The listing builds one solid part. Answer for the finished solid, in the listing's coordinates (mm). Give positions to 0.01 mm unless a question says otherwise; leave off trailing zeros. Order: outer loops, then holes, each group sorted by start corner. A loop starts at its lowest first (then second) coordinate and runs counter-clockwise, first axis right, second up.
```python
from build123d import *

# Parameters (mm, degrees)
SKETCH1_R           = 1.5875
BOSS_EXTRUDE1_DEPTH = 18.25625


with BuildPart() as part:
    # Sketch1 → Boss-Extrude1 (new body)
    with BuildSketch(Plane.XY):
        with BuildLine():
            Line((0, 990.6), (0, 0))
            Line((0, 0), (457.201, 0))
            Line((457.201, 0), (457.201, 13.862038208))
            ThreePointArc((457.201, 13.862038208), (232.767577124, 176.628269142), (124.367415652, 431.8))
            Line((124.367415652, 431.8), (50.8, 990.6))
            Line((50.8, 990.6), (0, 990.6))
        make_face()
        with Locations((18.25625, 18.25625)):
            Circle(SKETCH1_R, mode=Mode.SUBTRACT)
        with Locations((18.25625, 43.65625)):
            Circle(SKETCH1_R, mode=Mode.SUBTRACT)
        with Locations((56.35625, 63.5)):
            Circle(SKETCH1_R, mode=Mode.SUBTRACT)
        with Locations((56.35625, 101.6)):
            Circle(SKETCH1_R, mode=Mode.SUBTRACT)
        with Locations((388.14375, 18.25625)):
            Circle(SKETCH1_R, mode=Mode.SUBTRACT)
        with Locations((18.25625, 972.34375)):
            Circle(SKETCH1_R, mode=Mode.SUBTRACT)
    extrude(amount=BOSS_EXTRUDE1_DEPTH)


solid = part.part
```
1) Find section B-B (y = 498.5). Write down the section's boundary in (x, z).
Geometry says:
outline: (0, 0) - (115.59, 0) - (115.59, 18.26) - (0, 18.26) - close
2) Straight lines are drawn through the part: probe 1 along Y at (x, z) = (246, 10); probe 2 along Y at (x, z) = (256, 16.75); probe 3 along X at (y, z) = (425.5, 4.75). For each, find the intervals that lie inside material, in ascending order.
Geometry says:
probe 1: y = 0 to 160.68
probe 2: y = 0 to 149.44
probe 3: x = 0 to 125.24
3) Given P1, Ø3, axis at x = 18.26, y = 972.34, coming from the -Z side; P2, Ø6, axis at y = 548.5, z = 12.5, coming from the +X side; P3, Ø4, axis at x = 224, z = 12.5, coming from the +Y side; P4, Ø1, axis at y = 326.5, z = 7.5, coming from the +X side, each flat-ended and moving along its own axis, determine where each tip first touches the part or whether it passes through.
Geometry says:
P1: passes through
P2: stops at x = 109.4
P3: stops at y = 190.63
P4: stops at x = 149.82
4) Find section C-C (x = 165). Write down the section's boundary in (y, z), then the cut area to 3 significant figures.
Geometry says:
outline: (0, 0) - (288.08, 0) - (288.08, 18.26) - (0, 18.26) - close
area: 5,260 mm2
5) Find section A-A (z = 7). Write down the section's boundary in (x, y) (1 decimal).
Geometry says:
outline: (0, 0) - (457.2, 0) - (457.2, 13.9) arc R518.2 cw to (124.4, 431.8) - (50.8, 990.6) - (0, 990.6) - close; hole circle Ø3.2 at (18.3, 18.3); hole circle Ø3.2 at (18.3, 43.7); hole circle Ø3.2 at (18.3, 972.3); hole circle Ø3.2 at (56.4, 63.5); hole circle Ø3.2 at (56.4, 101.6); hole circle Ø3.2 at (388.1, 18.3)
